Answer from the drawing. Dimensions are ordinates in mm from the lowest x, y and z of the part. A direction names the side the tool comes from. Round coordinates to 2 decimals unless told otherwise and drop trailing zeros. Write each loop counter-clockwise with the first axis right and the second up, starting at its lowest first coordinate (ties: lowest second). Pieces come first, ordered by that corner, then holes. Notation, with made-up numbers: (-34.75, -10) - (-10.75, -10) arc R25 cw to (-10.75, 3) - close; hole circle Ø10 at (25, 50.25). An arc over 180 degrees is marked (long way). Answer as a JSON object with one key per item and string values.
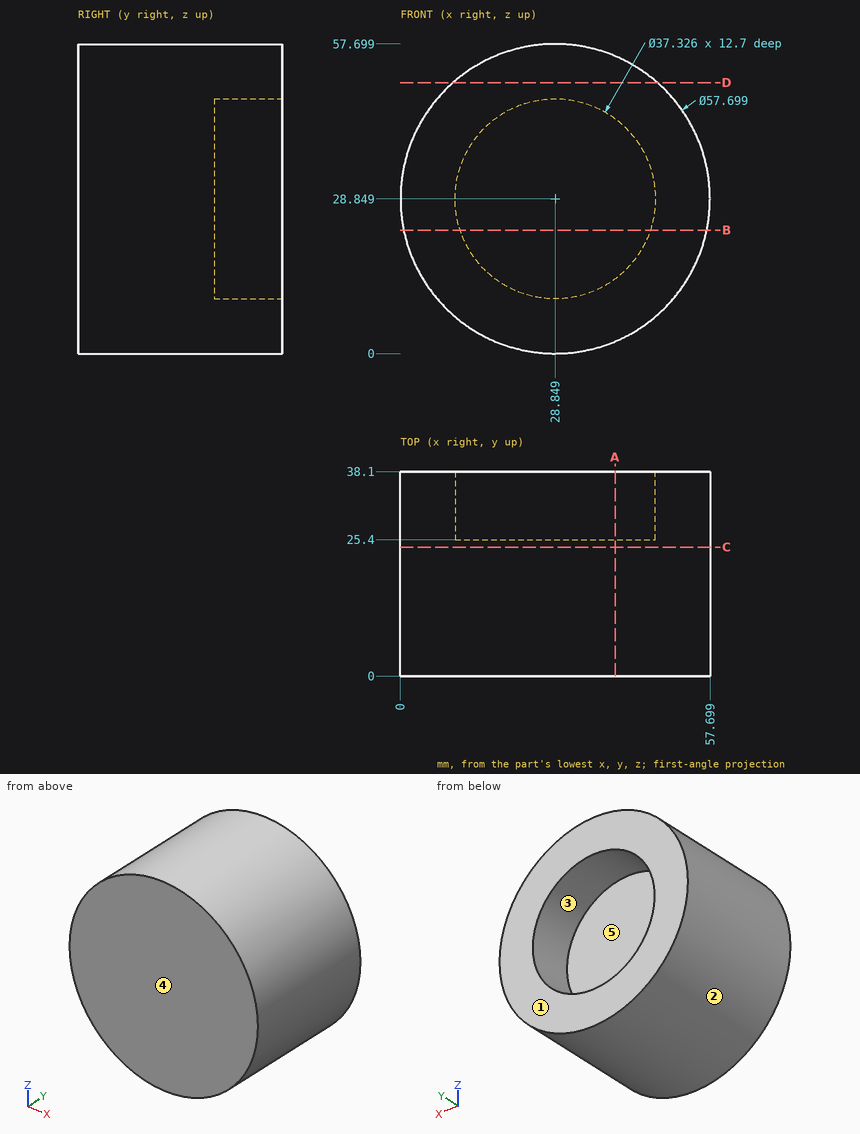
Item 1: For the marked faces 4 and 5, determine the directions among +Z, -Z, +X, -X, +Y, -Y from which every point of the face is accessible in a straight line to the end or side of a thin tool.
Results found:
{"face 4": "+Z, -Z, +X, -X, -Y", "face 5": "+Y"}
Item 2: A cutting plane is placed at B-B (z = 23). Write down the section's boundary in (x, y), and give its area (3 significant figures).
Results found:
{"outline": "(0.6, 0) - (57.1, 0) - (57.1, 38.1) - (46.57, 38.1) - (46.57, 25.4) - (11.13, 25.4) - (11.13, 38.1) - (0.6, 38.1) - close", "area": "1,700 mm²"}
Item 3: Consider line 1 along Z through (x, y) = (40, 29) (1 decimal); line 2 along Y through (x, z) = (18, 16); line 3 along X through (y, z) = (9, 28). Determine where each line is inside the solid, lowest interval first.
Results found:
{"line 1": "2.2 to 13.9, 43.8 to 55.5", "line 2": "0 to 25.4", "line 3": "0.01 to 57.69"}
Item 4: A cutting plane is placed at C-C (y = 24). Write down the section's boundary in (x, z).
Results found:
{"outline": "circle Ø57.7 at (28.85, 28.85)"}
Item 5: Determine the mould class of the marked faces 1, 2 and 3 for opening direction Z: pulls with the +Z half, pulls with the -Z half, needs draft (parallel to the pull), parting line crosses it, or undercut.
Results found:
{"face 1": "needs draft", "face 2": "parting line crosses it", "face 3": "undercut"}
Item 6: A cutting plane is placed at A-A (x = 40). Write down the section's boundary in (y, z) (1 decimal).
Results found:
{"outline": "(0, 2.2) - (38.1, 2.2) - (38.1, 13.9) - (25.4, 13.9) - (25.4, 43.8) - (38.1, 43.8) - (38.1, 55.5) - (0, 55.5) - close"}
Item 7: A cutting plane is placed at D-D (z = 50.5). Write down the section's boundary in (x, y) (1 decimal).
Results found:
{"outline": "(9.8, 0) - (47.9, 0) - (47.9, 38.1) - (9.8, 38.1) - close"}
Item 8: Each of these flat-tipped pins is pushed along its axis until it touches: P1, Ø6, axis at x = 15, z = 27.5, coming from the +Y side; P2, Ø3, axis at x = 35.5, y = 4, coming from the +Z side (1 decimal); P3, Ø5, axis at y = 28.5, z = 20.5, coming from the +X side. Where does it stop, or does it pass through?
Results found:
{"P1": "y = 25.4", "P2": "z = 57.2", "P3": "x = 57.1"}
